The model under review builds one solid part; all positions refer to its coordinate system, in mm. Face numbers are marked on the shaded views. A direction names the side the tool comes from. Round coordinates to 2 decimals unless told otherwise and drop trailing zeros. Write each loop counter-clockwise with the first axis right and the second up, starting at its lowest first coordinate (ties: lowest second). Pieces come first, ordered by that corner, then holes. Notation, with made-up numbers: (-3.5, 3) -> (42.5, 3) arc R32 ccw to (42.5, 29) -> close; hole circle Ø4 at (47.5, 64.5). An arc over 180 degrees is marked (long way). Answer as a JSON object with one key per item and string values. Group by question number.
1) Insertion check: pin 1 Ø24.5 at (x, y) = (-6, -1.5) entering from -Z; pin 2 Ø2 at (x, z) = (-3.5, 6) entering from +Y; pin 3 Ø5.5 at (x, y) = (0, 0) entering from +Z; pin 4 Ø4 at (x, y) = (-5.65, 5.65) entering from -Z. Each pin has a flat end and moves straight along its axis. Give the tip position at first contact, or say it passes through.
2) Machinability: for the marked faces 4 and 5, which of the approach directions +Z, -Z, +X, -X, +Y, -Y give a long, thin tool a straight path to every point of the face, cutting with its end or side? Answer none if there is none.
3) Mouldability with a two-part tool opening along Y and no side actions: class the marked faces 1, 2 and 3 as pulls with the +Y half, pulls with the -Y half, needs draft (parallel to the pull), parting line crosses it, or undercut.
4) To check wall thickness, follow probe 1 along Y at (x, z) = (18, 4.5); probe 2 along Y at (x, z) = (-5.65, 13.95); probe 3 along X at (y, z) = (20, 3.5). State the ranges of each line that lie inside material, in increasing order. Write a range as [from, to].
5) We need section C-C, the plane x = 14. Write out the cut boundary in (y, z).
6) We need section A-A, the plane y = 0. Write out the cut boundary in (x, z).
7) We need section B-B, the plane z = 10.5. Write out the cut boundary in (x, y), then the cut area to 3 significant figures.
8) We need section D-D, the plane y = 10. Write out the cut boundary in (x, z).
from build123d import *

# Parameters (mm, degrees)
SKETCH_1_R          = 29
EXTRUDE_1_DEPTH     = 15
SKETCH_2_R          = 25
CUT_EXTRUDE_1_DEPTH = 13
CUT_EXTRUDE_2_REACH = 17
SKETCH_3_R          = 1.3
SKETCH_3_R_2        = 3
EXTRUDE_3_DEPTH     = 10


with BuildPart() as part:
    # 草图1 → 凸台-拉伸1 (new body)
    with BuildSketch(Plane.XY):
        Circle(SKETCH_1_R)
    extrude(amount=EXTRUDE_1_DEPTH)

    # 草图2 → 切除-拉伸1 (cut)
    with BuildSketch(Plane(origin=(0, 0, 0), x_dir=(-1, 0, 0), z_dir=(0, 0, -1))):
        Circle(SKETCH_2_R)
    extrude(amount=-CUT_EXTRUDE_1_DEPTH, mode=Mode.SUBTRACT)

    # 草图3 → 切除-拉伸2 (cut, up to next)
    with BuildSketch(Plane.XY.offset(15), mode=Mode.PRIVATE) as cut_extrude_2_sk1:
        with Locations((5.65, 5.65)):
            Circle(SKETCH_3_R)
    cut_extrude_2_tool1 = extrude(cut_extrude_2_sk1.sketch, amount=-CUT_EXTRUDE_2_REACH, mode=Mode.PRIVATE) & part.part
    add(cut_extrude_2_tool1.solids().sort_by_distance((5.65, 5.65, 15))[0], mode=Mode.SUBTRACT)
    # 草图3 → 切除-拉伸2 (cut, up to next)
    with BuildSketch(Plane.XY.offset(15), mode=Mode.PRIVATE) as cut_extrude_2_sk2:
        with Locations((5.65, -5.65)):
            Circle(SKETCH_3_R)
    cut_extrude_2_tool2 = extrude(cut_extrude_2_sk2.sketch, amount=-CUT_EXTRUDE_2_REACH, mode=Mode.PRIVATE) & part.part
    add(cut_extrude_2_tool2.solids().sort_by_distance((5.65, -5.65, 15))[0], mode=Mode.SUBTRACT)
    # 草图3 → 切除-拉伸2 (cut, up to next)
    with BuildSketch(Plane.XY.offset(15), mode=Mode.PRIVATE) as cut_extrude_2_sk3:
        with Locations((-5.65, -5.65)):
            Circle(SKETCH_3_R)
    cut_extrude_2_tool3 = extrude(cut_extrude_2_sk3.sketch, amount=-CUT_EXTRUDE_2_REACH, mode=Mode.PRIVATE) & part.part
    add(cut_extrude_2_tool3.solids().sort_by_distance((-5.65, -5.65, 15))[0], mode=Mode.SUBTRACT)
    # 草图3 → 切除-拉伸2 (cut, up to next)
    with BuildSketch(Plane.XY.offset(15), mode=Mode.PRIVATE) as cut_extrude_2_sk4:
        with Locations((-5.65, 5.65)):
            Circle(SKETCH_3_R)
    cut_extrude_2_tool4 = extrude(cut_extrude_2_sk4.sketch, amount=-CUT_EXTRUDE_2_REACH, mode=Mode.PRIVATE) & part.part
    add(cut_extrude_2_tool4.solids().sort_by_distance((-5.65, 5.65, 15))[0], mode=Mode.SUBTRACT)
    # 草图3 → 切除-拉伸2 (cut, up to next)
    with BuildSketch(Plane.XY.offset(15), mode=Mode.PRIVATE) as cut_extrude_2_sk5:
        Circle(SKETCH_3_R_2)
    cut_extrude_2_tool5 = extrude(cut_extrude_2_sk5.sketch, amount=-CUT_EXTRUDE_2_REACH, mode=Mode.PRIVATE) & part.part
    add(cut_extrude_2_tool5.solids().sort_by_distance((0, 0, 15))[0], mode=Mode.SUBTRACT)

    # 草图4 → 凸台-拉伸3 (add)
    with BuildSketch(Plane(origin=(0, 0, 13), x_dir=(-1, 0, 0), z_dir=(0, 0, -1))):
        with BuildLine():
            Line((3.475322722, 16.89629048), (5.036699597, 24.487377507))
            ThreePointArc((5.036699597, 24.487377507), (-0.382728828, 24.997070201), (-5.784012851, 24.321702147))
            Line((-5.784012851, 24.321702147), (-3.990968867, 16.781974482))
            ThreePointArc((-3.990968867, 16.781974482), (-0.264082892, 17.247978439), (3.475322722, 16.89629048))
        make_face()
        with BuildLine():
            Line((16.370278146, 5.438427476), (23.725040792, 7.881778951))
            ThreePointArc((23.725040792, 7.881778951), (21.4567334, 12.829987989), (18.171205497, 17.169953138))
            Line((18.171205497, 17.169953138), (12.538131793, 11.847267665))
            ThreePointArc((12.538131793, 11.847267665), (14.805146046, 8.852691712), (16.370278146, 5.438427476))
        make_face()
        with BuildLine():
            Line((12.894955424, -11.457863003), (18.688341195, -16.605598556))
            ThreePointArc((18.688341195, -16.605598556), (21.839462229, -12.167082212), (23.955218348, -7.151749009))
            Line((23.955218348, -7.151749009), (16.52910066, -4.934706816))
            ThreePointArc((16.52910066, -4.934706816), (15.069228938, -8.395286727), (12.894955424, -11.457863003))
        make_face()
        with BuildLine():
            Line((-3.475322722, -16.89629048), (-5.036699597, -24.487377507))
            ThreePointArc((-5.036699597, -24.487377507), (0.382728828, -24.997070201), (5.784012851, -24.321702147))
            Line((5.784012851, -24.321702147), (3.990968867, -16.781974482))
            ThreePointArc((3.990968867, -16.781974482), (0.264082892, -17.247978439), (-3.475322722, -16.89629048))
        make_face()
        with BuildLine():
            Line((-16.370278146, -5.438427476), (-23.725040792, -7.881778951))
            ThreePointArc((-23.725040792, -7.881778951), (-21.4567334, -12.829987989), (-18.171205497, -17.169953138))
            Line((-18.171205497, -17.169953138), (-12.538131793, -11.847267665))
            ThreePointArc((-12.538131793, -11.847267665), (-14.805146046, -8.852691712), (-16.370278146, -5.438427476))
        make_face()
        with BuildLine():
            Line((-12.894955424, 11.457863003), (-18.688341195, 16.605598556))
            ThreePointArc((-18.688341195, 16.605598556), (-21.839462229, 12.167082212), (-23.955218348, 7.151749009))
            Line((-23.955218348, 7.151749009), (-16.52910066, 4.934706816))
            ThreePointArc((-16.52910066, 4.934706816), (-15.069228938, 8.395286727), (-12.894955424, 11.457863003))
        make_face()
    extrude(amount=EXTRUDE_3_DEPTH)


solid = part.part
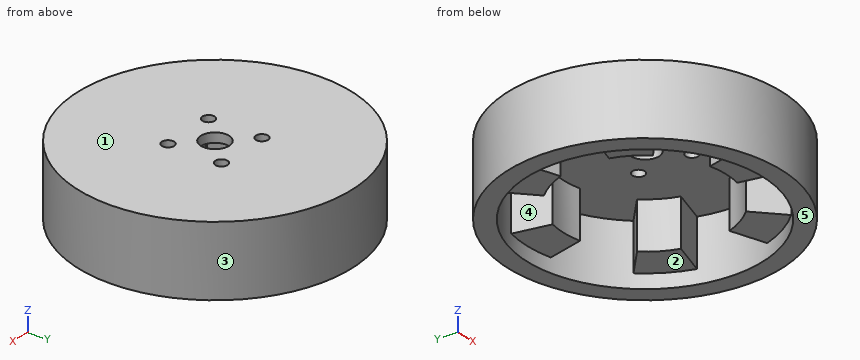
Here are the results:
{
 "1": {"pin 1": "stops at z = 3", "pin 2": "stops at y = 28.89", "pin 3": "passes through", "pin 4": "stops at z = 13"},
 "2": {"face 4": "-Z", "face 5": "-Z, +X, -X, +Y, -Y"},
 "3": {"face 1": "needs draft", "face 2": "undercut", "face 3": "parting line crosses it"},
 "4": {"probe 1": "y = [-22.74, -17.35], [-17.01, -5.98], [5.37, 15.99], [17.35, 22.74]", "probe 2": "y = [-28.44, -6.95], [-4.35, 4.35], [6.95, 28.44]", "probe 3": "x = [-21, -15], [-4.11, 4.76], [15, 21]"},
 "5": {"outline": "(-25.4, 0) -> (-20.71, 0) -> (-20.71, 13) -> (-13.23, 13) -> (-13.23, 3) -> (-10.08, 3) -> (-10.08, 13) -> (10.08, 13) -> (10.08, 3) -> (12.44, 3) -> (12.44, 13) -> (20.71, 13) -> (20.71, 0) -> (25.4, 0) -> (25.4, 15) -> (-25.4, 15) -> close"},
 "6": {"outline": "(-29, 0) -> (-25, 0) -> (-25, 13) -> (-3, 13) -> (-3, 15) -> (-29, 15) -> close; (3, 13) -> (25, 13) -> (25, 0) -> (29, 0) -> (29, 15) -> (3, 15) -> close"},
 "7": {"outline": "circle Ø58 at (0, 0); hole (-23.96, -7.15) -> (-16.53, -4.93) arc R17.25 ccw to (-12.89, -11.46) -> (-18.69, -16.61) arc R25 ccw to (-5.78, -24.32) -> (-3.99, -16.78) arc R17.25 ccw to (3.48, -16.9) -> (5.04, -24.49) arc R25 ccw to (18.17, -17.17) -> (12.54, -11.85) arc R17.25 ccw to (16.37, -5.44) -> (23.73, -7.88) arc R25 ccw to (23.96, 7.15) -> (16.53, 4.93) arc R17.25 ccw to (12.89, 11.46) -> (18.69, 16.61) arc R25 ccw to (5.78, 24.32) -> (3.99, 16.78) arc R17.25 ccw to (-3.48, 16.9) -> (-5.04, 24.49) arc R25 ccw to (-18.17, 17.17) -> (-12.54, 11.85) arc R17.25 ccw to (-16.37, 5.44) -> (-23.73, 7.88) arc R25 ccw to start", "area": "1,110 mm^2"},
 "8": {"outline": "(-27.22, 0) -> (-22.91, 0) -> (-22.91, 3) -> (-14.06, 3) -> (-14.06, 13) -> (14.06, 13) -> (14.06, 3) -> (22.91, 3) -> (22.91, 0) -> (27.22, 0) -> (27.22, 15) -> (-27.22, 15) -> close"}
}
